```python
from build123d import *

# Parameters (mm, degrees)
AUFSATZ_LINEAR_AUSTRAGEN1_OUTLINE_W                  = 30
AUFSATZ_LINEAR_AUSTRAGEN1_OUTLINE_H                  = 17
AUFSATZ_LINEAR_AUSTRAGEN1_DEPTH                      = 9
SKIZZE3_W                                            = 30
SKIZZE3_H                                            = 20
AUFSATZ_LINEAR_AUSTRAGEN2_DEPTH                      = 4
FASE1_SIZE                                           = 5
SKIZZE7_W                                            = 10
SKIZZE7_H                                            = 7
AUFSATZ_LINEAR_AUSTRAGEN3_DEPTH                      = 2
SCHNITT_LINEAR_AUSTRAGEN1_DEPTH                      = 45.206900067
LINEARES_MUSTER1_COUNT                               = 12
LINEARES_MUSTER1_PITCH                               = 0.5
AUFSATZ_LINEAR_START                                 = -5
AUFSATZ_LINEAR_AUSTRAGEN4_DEPTH                      = 10
SCHNITT_LINEAR_AUSTRAGEN2_DEPTH                      = 45.206900067
SCHNITT_LINEAR_AUSTRAGEN2_DEPTH_BACK                 = 45.206900067
SKIZZE10_W                                           = 5
SKIZZE10_H                                           = 4
AUFSATZ_LINEAR_AUSTRAGEN5_DEPTH                      = 2
SKIZZE13_W                                           = 5
SKIZZE13_H                                           = 4
SCHNITT_LINEAR_AUSTRAGEN3_DEPTH                      = 9
FASE2_SIZE                                           = 0.5
VERRUNDUNG1_R                                        = 1
STIRNSENKUNG_F_R_M4_ZYLINDERSCHRAUBE_MIT_D           = 4.5
STIRNSENKUNG_F_R_M4_ZYLINDERSCHRAUBE_MIT_CBORE_D     = 8
STIRNSENKUNG_F_R_M4_ZYLINDERSCHRAUBE_MIT_CBORE_DEPTH = 4.4
SKIZZE18_W                                           = 30
SKIZZE18_H                                           = 11
AUFSATZ_LINEAR_AUSTRAGEN6_DEPTH                      = 2
FASE3_SIZE                                           = 1


with BuildPart() as part:
    # Aufsatz-Linear austragen1: read off the stored shape, not the designer's step
    # Aufsatz-Linear austragen1 outline → Aufsatz-Linear austragen1 (new body)
    with BuildSketch(Plane.XY):
        Rectangle(AUFSATZ_LINEAR_AUSTRAGEN1_OUTLINE_W, AUFSATZ_LINEAR_AUSTRAGEN1_OUTLINE_H)
    extrude(amount=AUFSATZ_LINEAR_AUSTRAGEN1_DEPTH)

    # Skizze3 → Aufsatz-Linear austragen2 (add)
    with BuildSketch(Plane(origin=(0, 8.5, 0), x_dir=(1, 0, 0), z_dir=(0, 1, 0))):
        with Locations((0, 1)):
            Rectangle(SKIZZE3_W, SKIZZE3_H)
    extrude(amount=AUFSATZ_LINEAR_AUSTRAGEN2_DEPTH)

    # Skizze4 → Ausformung1 section 0
    with BuildSketch(Plane(origin=(0, 39.5, 0), x_dir=(1, 0, 0), z_dir=(0, 1, 0))):
        with BuildLine():
            Line((-5, 11), (5, 11))
            Line((5, 11), (5, 6))
            Line((5, 6), (-5, 6))
            Line((-5, 6), (-5, 11))
        make_face()
    # Skizze5 → Ausformung1 section 1
    with BuildSketch(Plane(origin=(0, 12.5, 0), x_dir=(1, 0, 0), z_dir=(0, 1, 0))):
        with BuildLine():
            Line((-5, 11), (5, 11))
            Line((5, 11), (5, -9))
            Line((5, -9), (-5, -9))
            Line((-5, -9), (-5, 11))
        make_face()
    loft()

    # Fase1
    fase1_edges = [part.edges().sort_by_distance(p)[0] for p in [
        (5, 12.5, -1),
        (-5, 12.5, -1),
    ]]
    chamfer(fase1_edges, length=FASE1_SIZE)

    # Skizze7 → Aufsatz-Linear austragen3 (add)
    with BuildSketch(Plane(origin=(0, 0, -11), x_dir=(-1, 0, 0), z_dir=(0, 0, -1))):
        with Locations((0, 36)):
            Rectangle(SKIZZE7_W, SKIZZE7_H)
    extrude(amount=AUFSATZ_LINEAR_AUSTRAGEN3_DEPTH)

    # Skizze6 → Schnitt-Linear austragen1 (cut, symmetric)
    with BuildSketch(Plane(origin=(0, 0, 0), x_dir=(0, 0, -1), z_dir=(1, 0, 0))):
        Polygon((13, 39), (12.5, 38.75), (13, 38.5), align=None)
    schnitt_linear_austragen1 = extrude(amount=SCHNITT_LINEAR_AUSTRAGEN1_DEPTH, both=True, mode=Mode.SUBTRACT)

    # Lineares Muster1: Schnitt-Linear austragen1 ×12
    with Locations(*[(0, -i * LINEARES_MUSTER1_PITCH, 0) for i in range(1, LINEARES_MUSTER1_COUNT)]):
        add(schnitt_linear_austragen1, mode=Mode.SUBTRACT)

    # Skizze8 → Aufsatz-Linear austragen4 (add)
    with BuildSketch(Plane(origin=(0, 0, 0), x_dir=(0, 0, -1), z_dir=(1, 0, 0)).offset(AUFSATZ_LINEAR_START)):
        with BuildLine():
            ThreePointArc((11, 32.082575695), (11.978451782, 32.394531565), (13, 32.5))
            Line((13, 32.5), (11, 32.5))
            Line((11, 32.5), (11, 32.082575695))
        make_face()
        with BuildLine():
            Line((11, 22.917424305), (11, 22))
            Line((11, 22), (13, 22))
            Line((13, 22), (13, 22.5))
            ThreePointArc((13, 22.5), (11.978451782, 22.605468435), (11, 22.917424305))
        make_face()
    extrude(amount=AUFSATZ_LINEAR_AUSTRAGEN4_DEPTH)

    # Skizze9 → Schnitt-Linear austragen2 (cut, two sides: drawn at the far end of the back side and taken through both)
    with BuildSketch(Plane(origin=(0, 0, 0), x_dir=(0, 0, -1), z_dir=(1, 0, 0)).offset(-SCHNITT_LINEAR_AUSTRAGEN2_DEPTH_BACK)):
        with BuildLine():
            Line((11, 32.082575695), (11, 22.917424305))
            ThreePointArc((11, 22.917424305), (8, 27.5), (11, 32.082575695))
        make_face()
    extrude(amount=SCHNITT_LINEAR_AUSTRAGEN2_DEPTH + SCHNITT_LINEAR_AUSTRAGEN2_DEPTH_BACK, mode=Mode.SUBTRACT)

    # Skizze10 → Aufsatz-Linear austragen5 (add)
    with BuildSketch(Plane(origin=(0, 0, -11), x_dir=(-1, 0, 0), z_dir=(0, 0, -1))):
        with Locations((2.5, 20)):
            Rectangle(SKIZZE10_W, SKIZZE10_H)
    extrude(amount=AUFSATZ_LINEAR_AUSTRAGEN5_DEPTH)

    # Skizze12 → Ausformung2 section 0
    with BuildSketch(Plane(origin=(0, 0, -21), x_dir=(-1, 0, 0), z_dir=(0, 0, -1))):
        with BuildLine():
            Line((0.5, 21), (4.5, 21))
            Line((4.5, 21), (4.5, 19))
            Line((4.5, 19), (0.5, 19))
            Line((0.5, 19), (0.5, 21))
        make_face()
    # Skizze11 → Ausformung2 section 1
    with BuildSketch(Plane(origin=(0, 0, -13), x_dir=(-1, 0, 0), z_dir=(0, 0, -1))):
        with BuildLine():
            Line((0, 18), (5, 18))
            Line((5, 18), (5, 22))
            Line((5, 22), (0, 22))
            Line((0, 22), (0, 18))
        make_face()
    loft()

    # Skizze13 → Schnitt-Linear austragen3 (cut)
    with BuildSketch(Plane(origin=(0, 0, -13), x_dir=(-1, 0, 0), z_dir=(0, 0, -1))):
        with Locations((-2.5, 20)):
            Rectangle(SKIZZE13_W, SKIZZE13_H)
    extrude(amount=-SCHNITT_LINEAR_AUSTRAGEN3_DEPTH, mode=Mode.SUBTRACT)

    # Fase2
    # the kernel refuses this chamfer: 0.5 mm, written as the material it takes off along each edge
    with BuildSketch(Plane(origin=(-6.359313388, 22.5, -13), x_dir=(0, 0.05286907949936605, 0.9986014522485384), z_dir=(1, 0, 0))) as fase2_piece_1:
        with BuildLine():
            Line((0.528690795, 0), (-FASE2_SIZE * 0.0528690794994, FASE2_SIZE * 0.998601452249))
            Line((-FASE2_SIZE * 0.0528690794994, FASE2_SIZE * 0.998601452249), (0, 0))
            ThreePointArc((0, 0), (0.271800807, 0.00698718), (0.528690795, 0))
        make_face()
    extrude(amount=12.718626777, mode=Mode.SUBTRACT)

    # Verrundung1
    # the kernel refuses this fillet: 1 mm, written as the material it takes off along each edge
    with BuildSketch(Plane(origin=(5, 27.5, -13), x_dir=(0, -0.9230106794344456, -0.38477433080958384), z_dir=(0, 0.38477433080958384, -0.9230106794344456))) as verrundung1_piece_1:
        with BuildLine():
            CenterArc((5 + VERRUNDUNG1_R, VERRUNDUNG1_R), VERRUNDUNG1_R, 180, 90)
            Line((5, VERRUNDUNG1_R), (5, 0))
            Line((5, 0), (5 + VERRUNDUNG1_R, 0))
        make_face()
    revolve(axis=Axis((5, 27.5, -13), (-1, 0, 0)), revolution_arc=231.320638443, mode=Mode.SUBTRACT)
    with BuildSketch(Plane(origin=(-5, 27.5, -13), x_dir=(0, 0.8772223630986392, -0.4800842901820881), z_dir=(0, -0.4800842901820881, -0.8772223630986392))) as verrundung1_piece_2:
        with BuildLine():
            CenterArc((5 + VERRUNDUNG1_R, VERRUNDUNG1_R), VERRUNDUNG1_R, 180, 90)
            Line((5, VERRUNDUNG1_R), (5, 0))
            Line((5, 0), (5 + VERRUNDUNG1_R, 0))
        make_face()
    revolve(axis=Axis((-5, 27.5, -13), (1, 0, 0)), revolution_arc=231.320638443, mode=Mode.SUBTRACT)

    # Stirnsenkung für M4 Zylinderschraube mit Innensechskant1 (through all)
    with Locations(Plane.XY.offset(9)):
        with Locations((-10.5, -1), (10.5, -1)):
            CounterBoreHole(STIRNSENKUNG_F_R_M4_ZYLINDERSCHRAUBE_MIT_D / 2, STIRNSENKUNG_F_R_M4_ZYLINDERSCHRAUBE_MIT_CBORE_D / 2, STIRNSENKUNG_F_R_M4_ZYLINDERSCHRAUBE_MIT_CBORE_DEPTH)

    # Skizze18 → Aufsatz-Linear austragen6 (add)
    with BuildSketch(Plane.XZ.offset(-8.5)):
        with Locations((0, -5.5)):
            Rectangle(SKIZZE18_W, SKIZZE18_H)
    extrude(amount=AUFSATZ_LINEAR_AUSTRAGEN6_DEPTH)

    # Fase3
    fase3_edges = [part.edges().sort_by_distance(p)[0] for p in [
        (-15, -1, 0),
        (15, -1, 0),
        (15, 6.5, -5.5),
        (-15, 6.5, -5.5),
        (0, 6.5, -11),
        (15, 12.5, -1),
        (-15, 12.5, -1),
    ]]
    chamfer(fase3_edges, length=FASE3_SIZE)


solid = part.part
```
Part model, mm, in its own coordinate system. A direction names the side the tool comes from. Round coordinates to 2 decimals unless told otherwise and drop trailing zeros. Loops run counter-clockwise (first coordinate to the right, second up) from the corner with the lowest first, then second, coordinate; pieces in that order, holes last. Notation, with made-up numbers: (66.5, 88) -> (102.5, 88) arc R8 cw to (102.5, 94) -> close; hole circle Ø10 at (-16, 87). An arc over 180 degrees is marked (long way). Use one line per item in the form item = value. Start each with the question number.
Item 1: Two-plate mould, pull along Y, no slides. Class faces 1 (the flat face through (12, -3, 4.6)), 2 (the flat face through (3, 18, -8)), 3 (the flat face through (5, 29, -3)), 4 (the flat face through (-14.5, 12, -0.9)): released by +Y, released by -Y, zero draft, split by the parting line, or undercut.
Item 2: Tool access for faces 5 (the flat face through (3, 20, -4)), 6 (the flat face through (-5, 26, -5)), 7 (the flat face through (12, 12.5, -1)): list every direction of +Z, -Z, +X, -X, +Y, -Y with a clear straight run to the whole face (end or side of a thin tool).
Item 3: Drill centre lines: line 1 along Z through (x, y) = (7.5, 9.5); line 2 along X through (y, z) = (19.5, -3); line 3 along Y through (x, z) = (-10.5, 6.9). Where is each one in solid material? Low to high.
Item 4: Drop flat-ended pins along their axis: pin 1 Ø1.6 at (x, z) = (-3.5, -12) entering from -Y; pin 2 Ø6 at (x, y) = (5, 31) entering from +Z; pin 3 Ø7.5 at (x, y) = (-1.5, -4) entering from -Z. Give the stop position or say it passes through.
Item 5: Band-saw the part on A-A (x = -12). List the corners of the cut face in (y, z).
Data:
q1.face_1 = undercut
q1.face_2 = undercut
q1.face_3 = zero draft
q1.face_4 = released by +Y
q2.face_5 = -Z, +X
q2.face_6 = +Z, -Z, -X, +Y
q2.face_7 = +Z, -Z, +X, +Y
q3.line_1 = -11 to 9
q3.line_2 = -5 to 5
q3.line_3 = -8.5 to -5, 3 to 12.5
q4.pin_1 = 18
q4.pin_2 = 0.39
q4.pin_3 = 0
q5.outline = (-8.5, 0) -> (-2.68, 0) -> (-2.68, 4.6) -> (-4.71, 4.6) -> (-4.71, 9) -> (-8.5, 9) -> close; (0.68, 0) -> (6.5, 0) -> (6.5, -10) -> (7.5, -11) -> (12.5, -11) -> (12.5, 9) -> (2.71, 9) -> (2.71, 4.6) -> (0.68, 4.6) -> close
